Geometry: final body of the model. Coordinates: model frame, mm. A direction names the side the tool comes from. Give positions to 0.01 mm unless a question says otherwise; leave off trailing zeros. Write each loop counter-clockwise with the first axis right and the second up, starting at its lowest first coordinate (ties: lowest second). Pieces come first, ordered by that corner, then holes. Notation, with made-up numbers: (22.25, 38.5) -> (46.25, 38.5) arc R25 ccw to (46.25, 75.5) -> close; hole circle Ø2 at (-27.5, 86.5). An arc over 180 degrees is marked (long way). Answer as a JSON object with one key per item and string values. Group by question number.
(1) Set-up query: faces 1 (the face through (101, 100, -59)), 2 (the face through (102.547, 95, -52)). Return all of +Z, -Z, +X, -X, +Y, -Y with unobstructed straight access to the full face (end or side cutting, diameter ignored); none if empty.
(2) Material intervals for probe 1 along Y at (x, z) = (87.5, -52.75); probe 2 along Z at (x, y) = (100.25, 99.25); probe 3 along Z at (x, y) = (100, 98), sorted ascending.
(3) Section query C-C on y = 96.5. Output: boundary loops of the cut face in (x, z).
(4) Section query A-A on x = 101. Output: boundary loops of the cut face in (y, z).
(5) Draft query along Z for faces 3 (the face through (102.282, 97.972, -42.365)), 4 (the face through (84, 103, -43)), 5 (the face through (92, 95, -61.367)). Return one class per face: +Z half, -Z half, draft (parallel to the pull), parting line (faces both ways), or undercut.
(6) Section query B-B on z = -50.5. Output: boundary loops of the cut face in (x, y).
(7) Contact query for a flat-ended pin moving along its axis: pin 1 Ø6 at (x, z) = (89.5, -50) entering from +Y. Output: stop coordinate, or through.
(8) Section query D-D on x = 97.5. Output: boundary loops of the cut face in (y, z), plus the area to 3 significant figures.
from build123d import *

# Parameters (mm, degrees)
SKETCH066_W  = 20
SKETCH066_H  = 20
PAD025_DEPTH = 2
SKETCH067_R  = 1.25
PAD026_DEPTH = 4
SKETCH068_R  = 0.75
PAD027_DEPTH = 3


with BuildPart() as part:
    # Sketch066 → Pad025 (new body)
    with BuildSketch(Plane.XZ):
        with Locations((92.5474607125, -51.3671462774)):
            Rectangle(SKETCH066_W, SKETCH066_H)
    extrude(amount=PAD025_DEPTH)

    # Sketch067 (on Face5 of Pad025) → Pad026 (join)
    with BuildSketch(Plane(origin=(0, 0, 0), x_dir=(1, 0, 0), z_dir=(0, 1, 0))):
        with Locations((84.128586, 59.880451)):
            Circle(SKETCH067_R)
        with Locations((101.127403, 59.880451)):
            Circle(SKETCH067_R)
        with Locations((101.127403, 42.843773)):
            Circle(SKETCH067_R)
        with Locations((84.128586, 42.843773)):
            Circle(SKETCH067_R)
    extrude(amount=PAD026_DEPTH)

    # Sketch068 (on Face14 of Pad026) → Pad027 (join)
    with BuildSketch(Plane(origin=(0, 4, 0), x_dir=(1, 0, 0), z_dir=(0, 1, 0))):
        with Locations((84.117188, 59.896854)):
            Circle(SKETCH068_R)
        with Locations((101.122879, 59.897358)):
            Circle(SKETCH068_R)
        with Locations((101.130592, 42.899231)):
            Circle(SKETCH068_R)
        with Locations((84.133583, 42.881302)):
            Circle(SKETCH068_R)
    extrude(amount=PAD027_DEPTH)


with BuildPart() as part_1:
    # Body009 placement: moved
    add(part.part.moved(Location((0, 96, 0))))


solid = part_1.part
Answer list:
{
 "1": {"face 1": "+Y", "face 2": "+Z, -Z, +X, +Y, -Y"},
 "2": {"probe 1": "94 to 96", "probe 2": "-60.77 to -58.99, -43.73 to -41.95", "probe 3": "-60.42 to -59.34, -43.38 to -42.3"},
 "3": {"outline": "circle Ø2.5 at (84.13, -59.88); circle Ø2.5 at (84.13, -42.84); circle Ø2.5 at (101.13, -59.88); circle Ø2.5 at (101.13, -42.84)"},
 "4": {"outline": "(94, -61.37) -> (96, -61.37) -> (96, -61.12) -> (100, -61.12) -> (100, -60.64) -> (103, -60.64) -> (103, -59.16) -> (100, -59.16) -> (100, -58.64) -> (96, -58.64) -> (96, -44.09) -> (100, -44.09) -> (100, -43.64) -> (103, -43.64) -> (103, -42.16) -> (100, -42.16) -> (100, -41.6) -> (96, -41.6) -> (96, -41.37) -> (94, -41.37) -> close"},
 "5": {"face 3": "undercut", "face 4": "draft", "face 5": "-Z half"},
 "6": {"outline": "(82.55, 94) -> (102.55, 94) -> (102.55, 96) -> (82.55, 96) -> close"},
 "7": {"pin 1": "y = 96"},
 "8": {"outline": "(94, -61.37) -> (96, -61.37) -> (96, -41.37) -> (94, -41.37) -> close", "area": "40.0 mm2"}
}
